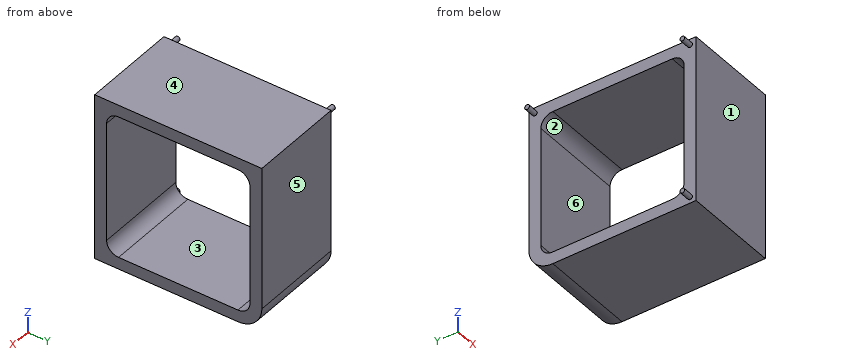
from build123d import *

# Parameters (mm, degrees)
EXTRUDE_1_DEPTH = 80
SKETCH_2_R      = 2
EXTRUDE_2_DEPTH = 9


with BuildPart() as part:
    # 草图1 → 凸台-拉伸1 (new body)
    with BuildSketch(Plane(origin=(0, 0, 0), x_dir=(0, 0, -1), z_dir=(1, 0, 0))):
        with BuildLine():
            Line((0, 0), (140, 0))
            Line((140, 0), (140, 120))
            ThreePointArc((140, 120), (134.142135624, 134.142135624), (120, 140))
            Line((120, 140), (0, 140))
            Line((0, 140), (0, 0))
        make_face()
        with BuildLine():
            Line((20, 130), (120, 130))
            ThreePointArc((120, 130), (127.071067812, 127.071067812), (130, 120))
            Line((130, 120), (130, 20))
            ThreePointArc((130, 20), (127.071067812, 12.928932188), (120, 10))
            Line((120, 10), (20, 10))
            ThreePointArc((20, 10), (12.928932188, 12.928932188), (10, 20))
            Line((10, 20), (10, 120))
            ThreePointArc((10, 120), (12.928932188, 127.071067812), (20, 130))
        make_face(mode=Mode.SUBTRACT)
    extrude(amount=EXTRUDE_1_DEPTH)

    # 草图2 → 凸台-拉伸2 (add)
    with BuildSketch(Plane.ZY):
        with Locations((-5, 135)):
            Circle(SKETCH_2_R)
        with Locations((-135, 5)):
            Circle(SKETCH_2_R)
        with Locations((-5, 5)):
            Circle(SKETCH_2_R)
    extrude(amount=EXTRUDE_2_DEPTH)


solid = part.part
For this review, take the finished solid that the model builds, in its own axes (mm). Face numbers are marked on the shaded views. A direction names the side the tool comes from. Give positions to 0.01 mm unless a question says otherwise; leave off trailing zeros. Order: outer loops, then holes, each group sorted by start corner. A loop starts at its lowest first (then second) coordinate and runs counter-clockwise, first axis right, second up. Notation, with made-up numbers: (5, -26) -> (32, -26) arc R23 cw to (32, 10) -> close; hole circle Ø3 at (64.5, 7.25). An arc over 180 degrees is marked (long way). Write item = value, one per line.
1) Draft analysis for pull direction Z (two halves, no side actions). For the marked faces 3, 4, 5 and 6, state which applies: pulls with the +Z half, pulls with the -Z half, needs draft (parallel to the pull), parting line crosses it, or undercut.
Findings:
face_3 = undercut
face_4 = pulls with the +Z half
face_5 = needs draft
face_6 = undercut
2) We need section C-C, the plane x = 9.5. Give the boundary of the cut face in (y, z).
Findings:
outline = (0, -140) -> (120, -140) arc R20 ccw to (140, -120) -> (140, 0) -> (0, 0) -> close; hole (10, -120) arc R10 ccw to (20, -130) -> (120, -130) arc R10 ccw to (130, -120) -> (130, -20) arc R10 ccw to (120, -10) -> (20, -10) arc R10 ccw to (10, -20) -> close
3) To check wall thickness, follow L1, parallel to Z at x = 9.5, y = 119; L2, parallel to Y at x = 52, z = -75; L3, parallel to X at y = 7, z = -7. State the ranges of each line that lie inside material, in increasing order. Write a range as from..to.
Findings:
L1 = -140..-130, -10..0
L2 = 0..10, 130..140
L3 = 0..80
4) We need section A-A, the plane z = -102. Give the boundary of the cut face in (x, y), and give its area (3 significant figures).
Findings:
outline = (0, 0) -> (80, 0) -> (80, 10) -> (0, 10) -> close; (0, 130) -> (80, 130) -> (80, 140) -> (0, 140) -> close
area = 1,600 mm^2
5) For the marked faces 1 and 2, list the 3-axis set-ups (+Z, -Z, +X, -X, +Y, -Y) from which the entire face can be reached by the end or side of a thin tool; tool diameter is ignored.
Findings:
face_1 = +Z, -Z, +X, -X, -Y
face_2 = +X, -X
6) Insertion check: pin 1 (1 mm diameter, centred on x = 67, y = 59, fed in from +Z). The pin has a flat end and moves straight along its axis. Give the tip position at first contact, or say it passes through.
Findings:
pin_1 = 0
7) We need section D-D, the plane z = -5. Give the boundary of the cut face in (x, y).
Findings:
outline = (-9, 3) -> (0, 3) -> (0, 0) -> (80, 0) -> (80, 140) -> (0, 140) -> (0, 137) -> (-9, 137) -> (-9, 133) -> (0, 133) -> (0, 7) -> (-9, 7) -> close
8) We need section B-B, the plane y = 70. Give the boundary of the cut face in (x, z), and give its area (3 significant figures).
Findings:
outline = (0, -140) -> (80, -140) -> (80, -130) -> (0, -130) -> close; (0, -10) -> (80, -10) -> (80, 0) -> (0, 0) -> close
area = 1,600 mm^2
